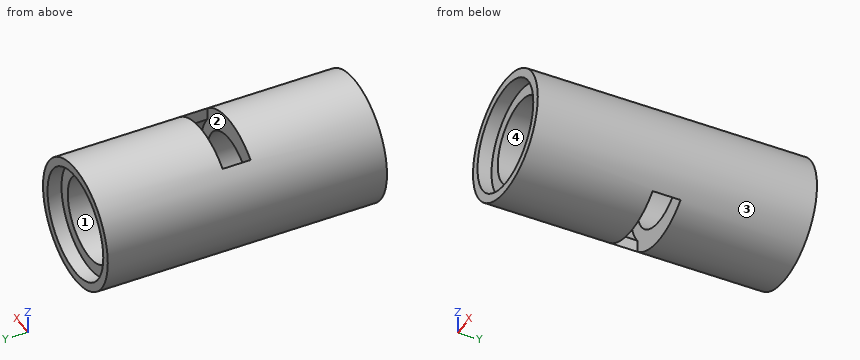
Solid Edge part; units mm, degrees
sketch "Sketch1" plane through (0, 0, 0) normal (0, -1, 0) x (1, 0, 0)
  circle A0 centre (0, 0) radius 3.6
extrude "Protrusion1" add sketch "Sketch1" against normal blind 16
sketch "Sketch2" plane through (0, 0, 0) normal (0, -1, 0) x (1, 0, 0)
  circle A0 centre (0, 0) radius 3.1
extrude "ExtrudedCutout_1" cut sketch "Sketch2" against normal blind 0.8
sketch "Sketch3" plane through (0, 16, 0) normal (0, 1, 0) x (-1, 0, 0)
  circle A0 centre (0, 0) radius 3.1
extrude "ExtrudedCutout_2" cut sketch "Sketch3" against normal blind 0.8
sketch "Sketch4" plane through (0, 0.8, 0) normal (0, -1, 0) x (1, 0, 0)
  circle A0 centre (0, 0) radius 2.4
extrude "ExtrudedCutout_3" cut sketch "Sketch4" against normal blind 20
sketch "Sketch5" plane through (0, 0, 0) normal (0, 0, 1) x (1, 0, 0)
  line L0 (-2, 8.8) -> (2, 8.8)
  line L1 (2, 8.8) -> (2.4, 8.8)
  line L2 (2.4, 8.8) -> (2.4, 7.2)
  line L3 (2.4, 7.2) -> (2, 7.2)
  line L4 (2, 7.2) -> (-2, 7.2)
  line L5 (-2.4, 7.2) -> (-2, 7.2)
  line L6 (-2.4, 8.8) -> (-2.4, 7.2)
  line L7 (-2, 8.8) -> (-2.4, 8.8)
extrude "ExtrudedCutout_5" cut sketch "Sketch5" along normal mid plane 60
sketch "Sketch6" plane through (0, 0, 0) normal (1, 0, 0) x (0, 1, 0)
  line L0 (8.8, 3.1) -> (8.8, 0)
  line L1 (7.2, 3.1) -> (7.2, 0)
  line L2 (8.8, 3.1) -> (7.2, 3.1)
revolve "RevolvedCutout1" cut sketch "Sketch6" angle 360 about axis through (0, 7.2, 0) along (0, 1, 0)
Could you check a few things on this model? Use its own coordinates, in mm. Face numbers are marked on the shaded views. A direction names the side the tool comes from. Coordinates: 2 decimals unless noted, no trailing zeros. Loops run counter-clockwise (first coordinate to the right, second up) from the corner with the lowest first, then second, coordinate; pieces in that order, holes last. Notation, with made-up numbers: (19, 36.5) -> (68, 36.5) arc R28 cw to (68, 68.5) -> close; hole circle Ø3 at (19, 37). An arc over 180 degrees is marked (long way). Answer in a Markdown table with one row per item.
(1) Will these pins go through, and if not, where does the flat tip stop? pin 1 Ø1.5 at (x, y) = (-2, 13) entering from +Z; pin 2 Ø0.8 at (y, z) = (7.5, -2.5) entering from +X; pin 3 Ø3 at (x, z) = (1, -0.5) entering from +Y.
Results found:
| item | result |
|---|---|
| pin 1 | stops at z = 3.38 |
| pin 2 | stops at x = 2.92 |
| pin 3 | stops at y = 15.2 |
(2) For the marked faces 1 and 2, which set-ups out of +Z, -Z, +X, -X, +Y, -Y let a thin tool reach every point of the face, with its end or its side?
Results found:
| item | result |
|---|---|
| face 1 | +Y, -Y |
| face 2 | none |
(3) Imagine slicing it at A-A (z = 0). List the corners of the cut face in (x, y) for me.
Results found:
| item | result |
|---|---|
| outline | (-3.6, 0) -> (-3.1, 0) -> (-3.1, 0.8) -> (-2.4, 0.8) -> (-2.4, 7.2) -> (-3.1, 7.2) -> (-3.1, 8.8) -> (-2.4, 8.8) -> (-2.4, 15.2) -> (-3.1, 15.2) -> (-3.1, 16) -> (-3.6, 16) -> close; (2.4, 0.8) -> (3.1, 0.8) -> (3.1, 0) -> (3.6, 0) -> (3.6, 16) -> (3.1, 16) -> (3.1, 15.2) -> (2.4, 15.2) -> (2.4, 8.8) -> (3.1, 8.8) -> (3.1, 7.2) -> (2.4, 7.2) -> close |
(4) If I drill on probe 1 along Y at (x, z) = (3, -0.5); probe 2 along Z at (x, y) = (0, 6); probe 3 along Z at (x, y) = (0, 0.45), over which ranges is the centre line in solid material (lowest first)?
Results found:
| item | result |
|---|---|
| probe 1 | y = 0.8 to 7.2, 8.8 to 15.2 |
| probe 2 | z = -3.6 to -2.4, 2.4 to 3.6 |
| probe 3 | z = -3.6 to -3.1, 3.1 to 3.6 |
(5) Imagine slicing it at D-D (x = -0.75). List the corners of the cut face in (y, z) for me.
Results found:
| item | result |
|---|---|
| outline | (0, -3.52) -> (7.2, -3.52) -> (7.2, -2.28) -> (0.8, -2.28) -> (0.8, -3.01) -> (0, -3.01) -> close; (0, 3.01) -> (0.8, 3.01) -> (0.8, 2.28) -> (7.2, 2.28) -> (7.2, 3.52) -> (0, 3.52) -> close; (8.8, -3.52) -> (16, -3.52) -> (16, -3.01) -> (15.2, -3.01) -> (15.2, -2.28) -> (8.8, -2.28) -> close; (8.8, 2.28) -> (15.2, 2.28) -> (15.2, 3.01) -> (16, 3.01) -> (16, 3.52) -> (8.8, 3.52) -> close |
(6) Thinking about a two-plate mould opening in Z: for the marked faces 3 and 4, which applies, released by +Z, released by -Z, zero draft, split by the parting line, or undercut?
Results found:
| item | result |
|---|---|
| face 3 | split by the parting line |
| face 4 | undercut |
(7) Imagine slicing it at C-C (x = 0). List the corners of the cut face in (y, z) for me.
Results found:
| item | result |
|---|---|
| outline | (0, -3.6) -> (7.2, -3.6) -> (7.2, -2.4) -> (0.8, -2.4) -> (0.8, -3.1) -> (0, -3.1) -> close; (0, 3.1) -> (0.8, 3.1) -> (0.8, 2.4) -> (7.2, 2.4) -> (7.2, 3.6) -> (0, 3.6) -> close; (8.8, -3.6) -> (16, -3.6) -> (16, -3.1) -> (15.2, -3.1) -> (15.2, -2.4) -> (8.8, -2.4) -> close; (8.8, 2.4) -> (15.2, 2.4) -> (15.2, 3.1) -> (16, 3.1) -> (16, 3.6) -> (8.8, 3.6) -> close |
(8) Imagine slicing it at B-B (y = 7.5). List the corners of the cut face in (x, z) for me, plus the area to 3 significant figures.
Results found:
| item | result |
|---|---|
| outline | (-2.4, -2.68) -> (-2.4, -1.96) arc R3.1 cw to (-2.4, 1.96) -> (-2.4, 2.68) arc R3.6 ccw to start; (2.4, -2.68) arc R3.6 ccw to (2.4, 2.68) -> (2.4, 1.96) arc R3.1 cw to (2.4, -1.96) -> close |
| area | 5.17 mm^2 |
